The listing builds one solid part. Answer for the finished solid, in the listing's coordinates (mm). Face numbers are marked on the shaded views. A direction names the side the tool comes from. Coordinates: 2 decimals unless noted, no trailing zeros. Write each loop counter-clockwise with the first axis right and the second up, starting at its lowest first coordinate (ties: lowest second). Pieces come first, ordered by that corner, then holes.
from build123d import *

# Parameters (mm, degrees)
SKETCH006_W     = 14
SKETCH006_H     = 14
PAD002_DEPTH    = 3
POCKET004_DEPTH = 2
SKETCH008_R     = 0.9
POCKET005_DEPTH = 1.001
PAD_DEPTH       = 3
SKETCH010_W     = 12
SKETCH010_H     = 12
POCKET_DEPTH    = 2
FILLET_R        = 2


with BuildPart() as obj1:
    # Sketch006 → Pad002 (new body)
    with BuildSketch(Plane.XY):
        Rectangle(SKETCH006_W, SKETCH006_H)
    extrude(amount=PAD002_DEPTH)

    # Sketch007 → Pocket004 (cut)
    with BuildSketch(Plane.XY.offset(3)):
        with BuildLine():
            Line((-3, 7), (-3, 4.963869))
            ThreePointArc((-3, 4.963869), (-5.8, 0), (-3, -4.963869))
            Line((-3, -7), (-3, -4.963869))
            Line((3, -7), (-3, -7))
            Line((3, -4.963869), (3, -7))
            ThreePointArc((3, -4.963869), (5.8, 0), (3, 4.963869))
            Line((3, 7), (3, 4.963869))
            Line((-3, 7), (3, 7))
        make_face()
    extrude(amount=-POCKET004_DEPTH, mode=Mode.SUBTRACT)

    # Sketch008 → Pocket005 (cut, through all)
    with BuildSketch(Plane.XY.offset(1)):
        Circle(SKETCH008_R)
    extrude(amount=-POCKET005_DEPTH, mode=Mode.SUBTRACT)


with BuildPart() as corner_holder_single:
    # Sketch → Pad (new body)
    with BuildSketch(Plane.XY):
        Polygon((-7, -7), (-7, 7), (7, 7), (7, 5), (-5, -7), align=None)
    extrude(amount=PAD_DEPTH)

    # Sketch010 → Pocket (cut)
    with BuildSketch(Plane(origin=(0, 0, 0), x_dir=(1, 0, 0), z_dir=(0, 0, -1))):
        with Locations((1, 1)):
            Rectangle(SKETCH010_W, SKETCH010_H)
    extrude(amount=-POCKET_DEPTH, mode=Mode.SUBTRACT)


with BuildPart() as corner_holder_single_1:
    # Clone placement: moved
    add(corner_holder_single.part.moved(Location((14, 0, 0))))

    # Fusion: union obj1
    add(obj1.part)

    # Fillet
    fillet_edges = [corner_holder_single_1.edges().sort_by_distance(p)[0] for p in [
        (-7, -7, 1.5),
        (-7, 7, 1.5),
    ]]
    fillet(fillet_edges, radius=FILLET_R)


with BuildPart() as corner_holder_single_2:
    # Clone001004 placement: moved
    add(corner_holder_single_1.part.moved(Location((-35.64867, 51.755502, 0))))


solid = corner_holder_single_2.part
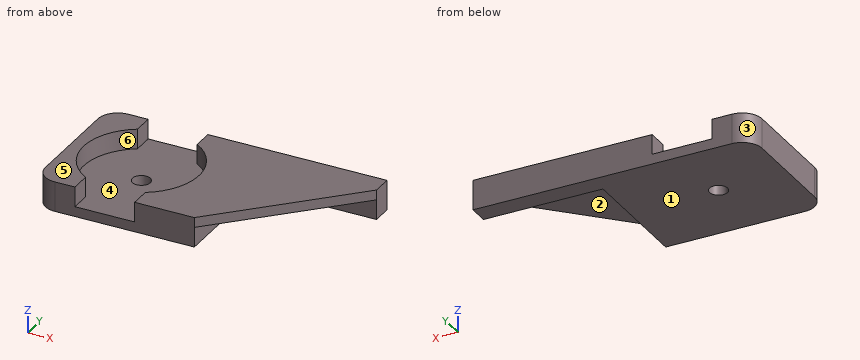
1. Section B-B on y = 51.25 is taken. Give the vertices of the cut face in (x, z), then the cut area to 3 significant figures.
Results found:
outline: (-42.65, 0) - (-36.39, 0) - (-36.39, 1) - (-41.43, 1) - (-41.43, 3) - (-42.65, 3) - close; (-34.9, 0) - (-26.65, 0) - (-26.65, 2) - (-20.15, 2) - (-20.15, 3) - (-29.87, 3) - (-29.87, 1) - (-34.9, 1) - close
area: 29.9 mm2
2. Section D-D on y = 53.5 is taken. Give the vertices of the cut face in (x, z), then the cut area to 3 significant figures.
Results found:
outline: (-42.65, 0) - (-26.65, 0) - (-26.65, 2) - (-17.9, 2) - (-17.9, 3) - (-30.12, 3) - (-30.12, 1) - (-41.18, 1) - (-41.18, 3) - (-42.65, 3) - close
area: 34.6 mm2
3. Flat-ended cylindrical pins translate along their axes: P1, Ø1.5, axis at y = 53, z = 1, coming from the +X side; P2, Ø0.6, axis at x = -22.5, z = 1, coming from the -Y side; P3, Ø1, axis at y = 45.5, z = 2, coming from the +X side. Find the tip coordinate at first contact, or state that the pin passes through.
Results found:
P1: stops at x = -26.65
P2: stops at y = 56.76
P3: stops at x = -25.4
4. A tool of negligible diameter and unlimited length cuts with its end or side. For the marked faces 1 and 2, from which of +Z, -Z, +X, -X, +Y, -Y can it reach the whole face along a straight path? Write none if from no direction.
Results found:
face 1: -Z, +X, -X, +Y, -Y
face 2: -Z, +X, -Y
5. For a pull along X with two mould halves and no side action, classify the marked faces 3, 4, 5 and 6 as pulls with the +X half, pulls with the -X half, needs draft (parallel to the pull), parting line crosses it, or undercut.
Results found:
face 3: pulls with the -X half
face 4: undercut
face 5: needs draft
face 6: undercut
6. Section A-A on z = 2.5 is taken. Give the vertices of the cut face in (x, y), then the cut area to 3 significant figures.
Results found:
outline: (-42.65, 46.76) arc R2 ccw to (-40.65, 44.76) - (-38.65, 44.76) - (-38.65, 46.79) arc R5.8 cw to (-38.65, 56.72) - (-38.65, 58.76) - (-40.65, 58.76) arc R2 ccw to (-42.65, 56.76) - close; (-32.65, 44.76) - (-26.65, 44.76) - (-14.65, 56.76) - (-14.65, 58.76) - (-32.65, 58.76) - (-32.65, 56.72) arc R5.8 cw to (-32.65, 46.79) - close
area: 195 mm2
7. Find the intervals of material crossed by L1, parallel to X at y = 51.5, z = 1.9; L2, parallel to Y at x = -18.25, z = 0.8; L3, parallel to Z at x = -21.25, y = 51.5, in increasing order.
Results found:
L1: x = -42.65 to -41.44, -29.85 to -26.65
L2: y = 56.76 to 58.76
L3: z = 2 to 3
8. Section C-C on x = -35.5 is taken. Give the vertices of the cut face in (y, z).
Results found:
outline: (44.76, 0) - (50.87, 0) - (50.87, 1) - (44.76, 1) - close; (52.64, 0) - (58.76, 0) - (58.76, 1) - (52.64, 1) - close
